Autodesk Inventor part; units mm, degrees
ref_plane "YZ Plane" through (0, 0, 0) normal (1, 0, 0) x (0, 1, 0)
ref_plane "XZ Plane" through (0, 0, 0) normal (0, 1, 0) x (-1, 0, 0)
ref_plane "XY Plane" through (0, 0, 0) normal (0, 0, 1) x (1, 0, 0)
sketch "Sketch1" plane through (0, 0, 0) normal (0, 1, 0) x (-1, 0, 0)
  line L0 (0, 0) -> (24, 0)
  line L1 (24, 0) -> (24, -48)
  line L2 (24, -48) -> (0, -48)
  line L3 (0, -48) -> (0, 0)
  line L4 (12, 0) -> (12, -48) construction
  circle A0 centre (12, -12) radius 9 construction
  dimension "d0" = 18
  dimension "d1" = 3
  dimension "d2" = 3
  dimension "d3" = 48
extrude "Extrusion1" add sketch "Sketch1" along normal blind 2
sketch "Sketch2" plane through (0, 2, 0) normal (0, 1, 0) x (1, 0, 0)
  line L0 (-24, 48) -> (-24, 0)
  line L1 (0, 0) -> (0, 48)
  line L2 (-24, 48) -> (0, 48)
  line L3 (0, 48) -> (0, 46)
  line L4 (0, 46) -> (-24, 46)
  line L5 (-24, 46) -> (-24, 48)
  dimension "d6" = 2
extrude "Extrusion2" add sketch "Sketch2" along normal blind 50
sketch "Sketch3" plane through (-24, 2, -46) normal (0, 0, 1) x (1, 0, 0)
  line L0 (24, 50) -> (0, 50) construction
  line L1 (12, 50) -> (12, 0) construction
  line L2 (0, 0) -> (24, 0) construction
  line L3 (12, 47) -> (12, 37) construction
  line L4 (9, 44) -> (9, 40)
  line L5 (15, 40) -> (15, 44)
  arc A0 (15, 44) -> (9, 44) centre (12, 44) ccw
  arc A1 (9, 40) -> (15, 40) centre (12, 40) ccw
  line L6 (12, 22) -> (12, 12) construction
  line L7 (9, 19) -> (9, 15)
  line L8 (15, 15) -> (15, 19)
  arc A2 (15, 19) -> (9, 19) centre (12, 19) ccw
  arc A3 (9, 15) -> (15, 15) centre (12, 15) ccw
  point P0 (24, -2)
  point P1 (12, 42)
  point P2 (12, 17)
  dimension "d9" = 6
  dimension "d10" = 10
  dimension "d11" = 3
  dimension "d12" = 10
  dimension "d13" = 6
  dimension "d14" = 15
extrude "Extrusion3" cut sketch "Sketch3" against normal up to next
sketch "Sketch4" plane through (0, 2, 0) normal (0, 1, 0) x (1, 0, 0)
  line L0 (-24, 0) -> (0, 0) construction
  line L1 (-12, 0) -> (-12, 46) construction
  line L2 (-9, 46) -> (-15, 46) construction
  circle A0 centre (-12, 11.5) radius 8.5
  dimension "d17" = 17
  dimension "d18" = 3
extrude "Extrusion4" add sketch "Sketch4" along normal blind 150
sketch "Sketch5" plane through (-12, 152, -11.5) normal (0, 1, 0) x (1, 0, 0)
  circle A0 centre (0, 0) radius 8.5
  circle A1 centre (0, 0) radius 20
  point P0 (12, -11.5)
  dimension "d21" = 40
extrude "Extrusion5" add sketch "Sketch5" along normal blind 95 contours A0 | A1
sketch "Sketch6" plane through (-12, 247, -11.5) normal (0, 1, 0) x (1, 0, 0)
  circle A0 centre (0, 0) radius 20
  circle A1 centre (0, 0) radius 19.9
  point P0 (12, -11.5)
  dimension "d24" = 0.1
sketch "Sketch6 outline for Extrusion6" plane through (-12, 247, -11.5) normal (0, 1, 0) x (1, 0, 0)
  circle A0 centre (0, 0) radius 19.9
extrude "Extrusion6" add sketch "Sketch6 outline for Extrusion6" along normal blind 59
sketch "Sketch7" plane through (-12, 306, -11.5) normal (0, 1, 0) x (1, 0, 0)
  circle A0 centre (0, 0) radius 19.9
  circle A1 centre (0, 0) radius 20
  point P0 (12, -11.5)
  dimension "d27" = 0.1
extrude "Extrusion7" add sketch "Sketch7" along normal blind 1 contours A0 | A1
sketch "Sketch8" plane through (-12, 307, -11.5) normal (0, 1, 0) x (1, 0, 0)
  circle A0 centre (0, 0) radius 19.9
  point P0 (12, -11.5)
extrude "Extrusion8" add sketch "Sketch8" along normal blind 59
sketch "Sketch9" plane through (-12, 366, -11.5) normal (0, 1, 0) x (1, 0, 0)
  circle A0 centre (0, 0) radius 19.9
  circle A1 centre (0, 0) radius 20
  point P0 (12, -11.5)
extrude "Extrusion9" add sketch "Sketch9" along normal blind 1 contours A0 | A1
sketch "Sketch10" plane through (-12, 367, -11.5) normal (0, 1, 0) x (1, 0, 0)
  circle A0 centre (0, 0) radius 19.9
  point P0 (12, -11.5)
extrude "Extrusion10" add sketch "Sketch10" along normal blind 59
sketch "Sketch11" plane through (-12, 426, -11.5) normal (0, 1, 0) x (1, 0, 0)
  circle A0 centre (0, 0) radius 20
  point P0 (12, -11.5)
extrude "Extrusion11" add sketch "Sketch11" along normal blind 10
fillet "Fillet1" radius 4 1 edges at (-32, 436, -11.5)
fillet "Fillet2" radius 5 1 edges at (-20.5, 152, -11.5)
equation "\"d2\" = d1"
properties part number "Signal Tower"
Can you work these out from the model? Positions are in its coordinate system, mm. A direction names the side the tool comes from. Give positions to 0.01 mm unless a question says otherwise; leave off trailing zeros. Write each loop counter-clockwise with the first axis right and the second up, starting at its lowest first coordinate (ties: lowest second). Pieces come first, ordered by that corner, then holes. Notation, with made-up numbers: M 35,88 L 93,88 A16 cw 93,103 Z; hole C -2,-10.75 d7. An arc over 180 degrees is marked long. Answer in a Markdown table with one row per item. Add a question column.
Item 1: Please list where these lines run through material, in increasing order: L1, parallel to Y at x = -20.5, z = 2; L2, parallel to Y at x = -1.5, z = -23.5; L3, parallel to Z at x = -10.5, y = 266.
Item 2: We'd pull the mould along Z, two halves only. Please class faces 1 (the flat face through (-12, 27, -46)), 2 (the cylindrical face through (-31.98, 198.84, -10.62)), 3 (the flat face through (-12, 0, -24)): released by +Z, released by -Z, zero draft, split by the parting line, or undercut.
Item 3: Imagine slicing it at A-A, the plane y = 174.5. Write out the boundary of the cut face in (x, z).
Item 4: For pin 1 Ø2 at (y, z) = (78, -12.5) entering from -X; pin 2 Ø2 at (y, z) = (43.5, -46.5) entering from +X; pin 3 Ø1 at (y, z) = (19, -47) entering from -X, each with a flat end and sliding along its axis, tell me the tip position at first contact or that it passes through.
Item 5: Imagine slicing it at B-B, the plane y = 409. Write out the boundary of the cut face in (x, z), plus the area to 3 significant figures.
Item 6: On a 3-axis mill with a long thin cutter (end or side, diameter ignored), from which of +Z, -Z, +X, -X, +Y, -Y can I reach the whole of each face in a straight line? I mean faces 4 (the flat face through (1, 152, -7)), 5 (the flat face through (0, 14, -47)), 6 (the flat face through (-24, 14, -47)). Say none if no direction works.
Evaluation:
| question | item | result |
|---|---|---|
| 1 | L1 | y = 152 to 436 |
| 1 | L2 | y = 0 to 2, 152 to 436 |
| 1 | L3 | z = -31.34 to 8.34 |
| 2 | face 1 | undercut |
| 2 | face 2 | split by the parting line |
| 2 | face 3 | zero draft |
| 3 | outline | C -12,-11.5 d40 |
| 4 | pin 1 | stops at x = -20.5 |
| 4 | pin 2 | stops at x = 0 |
| 4 | pin 3 | stops at x = -24 |
| 5 | outline | C -12,-11.5 d39.8 |
| 5 | area | 1,240 mm² |
| 6 | face 4 | none |
| 6 | face 5 | +Z, -Z, +X, -Y |
| 6 | face 6 | +Z, -Z, -X, -Y |
